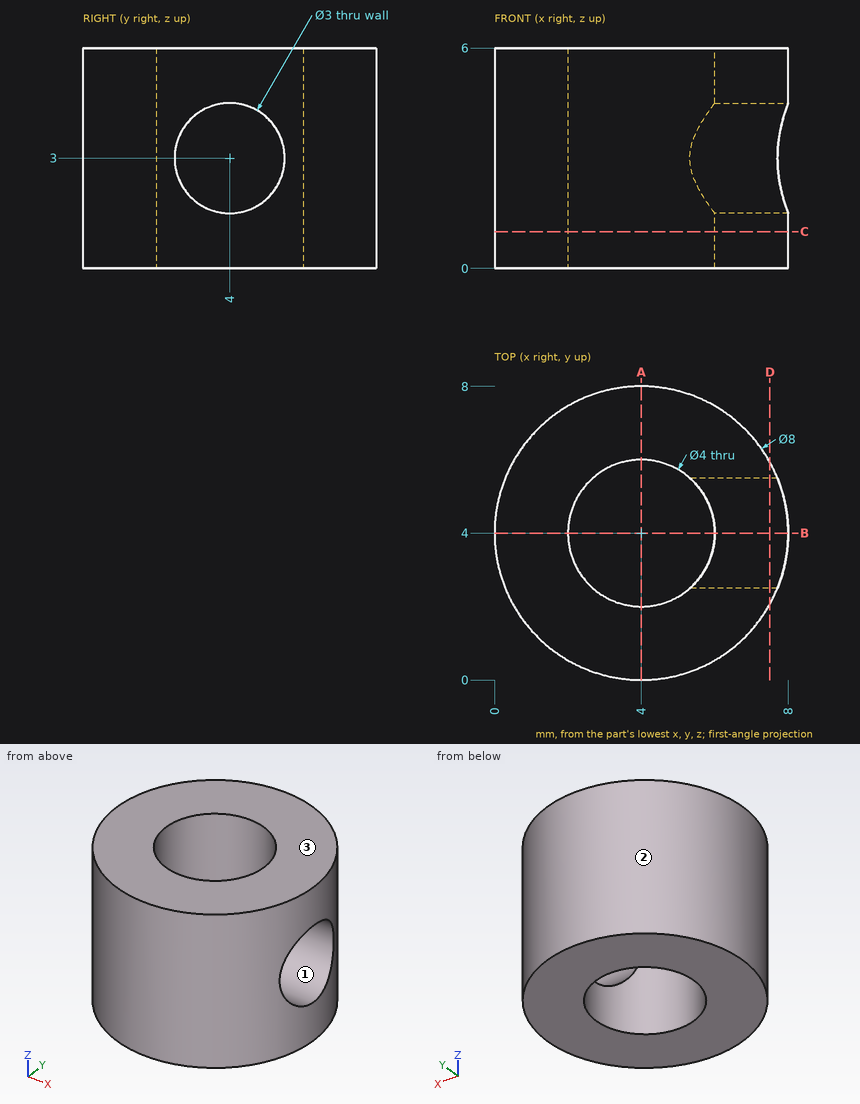
Job drawing, mm, ordinate dimensions from the low corner. One solid piece. Coordinates: 2 decimals unless noted, no trailing zeros. Order: outer loops, then holes, each group sorted by start corner. A loop starts at its lowest first (then second) coordinate and runs counter-clockwise, first axis right, second up. Notation, with made-up numbers: M 34,46.25 L 68,46.25 A9 ccw 68,58.25 Z; hole C 26,56 d5. An arc over 180 degrees is marked long. Answer as CSV lines item,"result".
(1) Band-saw the part on B-B, the plane y = 4. List the corners of the cut face in (x, z).
Geometry says:
outline,"M 0,0 L 2,0 L 2,6 L 0,6 Z; M 6,0 L 8,0 L 8,1.5 L 6,1.5 Z; M 6,4.5 L 8,4.5 L 8,6 L 6,6 Z"
(2) Band-saw the part on C-C, the plane z = 1. List the corners of the cut face in (x, y).
Geometry says:
outline,"C 4,4 d8; hole C 4,4 d4"
(3) Flat gauge pins, fed straight in: pin 1 (1 mm diameter, centred on x = 6.5, z = 4, fed in from -Y); pin 2 (3 mm diameter, centred on y = 3.5, z = 3.5, fed in from +X); pin 3 (2.5 mm diameter, centred on y = 4, z = 3, fed in from +X). Where does each tip first touch, or does it go through?
Geometry says:
pin 1,"stops at y = 0.54"
pin 2,"stops at x = 8"
pin 3,"stops at x = 2.44"
(4) Wall check: line 1 along X through (y, z) = (4.5, 5); line 2 along X through (y, z) = (3, 0.5); line 3 along Y through (x, z) = (4, 4.5). Give the ranges that are in metal, low to high.
Geometry says:
line 1,"x = 0.03 to 2.06, 5.94 to 7.97"
line 2,"x = 0.13 to 2.27, 5.73 to 7.87"
line 3,"y = 0 to 2, 6 to 8"
(5) Band-saw the part on A-A, the plane x = 4. List the corners of the cut face in (y, z).
Geometry says:
outline,"M 0,0 L 2,0 L 2,6 L 0,6 Z; M 6,0 L 8,0 L 8,6 L 6,6 Z"
(6) Band-saw the part on D-D, the plane x = 7.5. List the corners of the cut face in (y, z).
Geometry says:
outline,"M 2.06,0 L 5.94,0 L 5.94,6 L 2.06,6 Z; hole C 4,3 d3"
(7) Pull direction Y, two halves, no side cores. Call the marked faces 1, 2 and 3: +Y half, -Y half, draft (parallel to the pull), parting line (faces both ways), or undercut.
Geometry says:
face 1,"undercut"
face 2,"parting line"
face 3,"draft"
